Can you work these out from the model? Positions are in its coordinate system, mm. A direction names the side the tool comes from. Round coordinates to 2 decimals unless told otherwise and drop trailing zeros. Order: outer loops, then holes, each group sorted by start corner. A loop starts at its lowest first (then second) coordinate and runs counter-clockwise, first axis right, second up. Notation, with made-up numbers: (57, 22.5) -> (69, 22.5) arc R17 ccw to (69, 31.5) -> close; hole circle Ø7 at (34.25, 68). An arc over 180 degrees is marked (long way). One line per item, written item: value.
```python
from build123d import *

# Parameters (mm, degrees)
SKETCH1_W           = 45
SKETCH1_H           = 46
BOSS_EXTRUDE1_DEPTH = 30
SKETCH3_R           = 3.5
CUT_EXTRUDE2_DEPTH  = 10
SKETCH4_R           = 2.75
CUT_EXTRUDE3_DEPTH  = 59.77074102
SKETCH2_W           = 40
SKETCH2_H           = 40
CUT_EXTRUDE4_DEPTH  = 44.991476447


with BuildPart() as part:
    # Sketch1 → Boss-Extrude1 (new body)
    with BuildSketch(Plane(origin=(0, 0, 0), x_dir=(1, 0, 0), z_dir=(0, 1, 0))):
        Rectangle(SKETCH1_W, SKETCH1_H)
    extrude(amount=BOSS_EXTRUDE1_DEPTH)

    # Sketch3 → Cut-Extrude2 (cut)
    with BuildSketch(Plane(origin=(0, 0, -23), x_dir=(-1, 0, 0), z_dir=(0, 0, -1))):
        with Locations((0, 15)):
            Circle(SKETCH3_R)
    extrude(amount=-CUT_EXTRUDE2_DEPTH, mode=Mode.SUBTRACT)

    # Sketch4 → Cut-Extrude3 (cut, through all)
    with BuildSketch(Plane(origin=(22.5, 0, 0), x_dir=(0, 0, -1), z_dir=(1, 0, 0))):
        with Locations((0, 15)):
            Circle(SKETCH4_R)
    extrude(amount=-CUT_EXTRUDE3_DEPTH, mode=Mode.SUBTRACT)

    # Sketch2 → Cut-Extrude4 (cut, through all)
    with BuildSketch(Plane(origin=(0, 30, 0), x_dir=(1, 0, 0), z_dir=(0, 1, 0))):
        Rectangle(SKETCH2_W, SKETCH2_H)
    extrude(amount=-CUT_EXTRUDE4_DEPTH, mode=Mode.SUBTRACT)


solid = part.part
```
Q1. We'd pull the mould along X, two halves only. Please class faces 4 (the face through (22.5, 11, 0)), 5 (the face through (0, 11, -23)), 6 (the face through (0, 15, 20)), 7 (the face through (-22.5, 11, 0)): released by +X, released by -X, zero draft, split by the parting line, or undercut.
Answers below:
face 4: released by +X
face 5: zero draft
face 6: undercut
face 7: released by -X
Q2. I want a section at B-B on x = -4.5. List the corners of the cut face in (y, z) for me, plus the area to 3 significant figures.
Answers below:
outline: (0, -23) -> (30, -23) -> (30, -20) -> (0, -20) -> close; (0, 20) -> (30, 20) -> (30, 23) -> (0, 23) -> close
area: 180 mm^2
Q3. I want a section at C-C on y = 7.5. List the corners of the cut face in (x, z) for me, plus the area to 3 significant figures.
Answers below:
outline: (-22.5, -23) -> (22.5, -23) -> (22.5, 23) -> (-22.5, 23) -> close; hole (-20, -20) -> (20, -20) -> (20, 20) -> (-20, 20) -> close
area: 470 mm^2
Q4. I want a section at A-A on z = 0. List the corners of the cut face in (x, y) for me.
Answers below:
outline: (-22.5, 0) -> (-20, 0) -> (-20, 12.25) -> (-22.5, 12.25) -> close; (-22.5, 17.75) -> (-20, 17.75) -> (-20, 30) -> (-22.5, 30) -> close; (20, 0) -> (22.5, 0) -> (22.5, 12.25) -> (20, 12.25) -> close; (20, 17.75) -> (22.5, 17.75) -> (22.5, 30) -> (20, 30) -> close
Q5. Please list where these lines run through material, in increasing order: line 1 along X through (y, z) = (20.75, -16); line 2 along Z through (x, y) = (-11.5, 9); line 3 along Y through (x, z) = (0, -22.3).
Answers below:
line 1: -22.5 to -20, 20 to 22.5
line 2: -23 to -20, 20 to 23
line 3: 0 to 11.5, 18.5 to 30
Q6. On a 3-axis mill with a long thin cutter (end or side, diameter ignored), from which of +Z, -Z, +X, -X, +Y, -Y can I reach the whole of each face in a straight line? I mean faces 1 (the face through (-22, 30, 0)), 2 (the face through (0, 19, -20)), 3 (the face through (0.759, 11.583, -21.521)). Say none if no direction works.
Answers below:
face 1: +Z, -Z, +X, -X, +Y
face 2: +Y, -Y
face 3: -Z
Q7. I want a section at D-D on x = 0. List the corners of the cut face in (y, z) for me.
Answers below:
outline: (0, -23) -> (11.5, -23) -> (11.5, -20) -> (0, -20) -> close; (0, 20) -> (30, 20) -> (30, 23) -> (0, 23) -> close; (18.5, -23) -> (30, -23) -> (30, -20) -> (18.5, -20) -> close
